Design review of the part shown in the three views and the two pictorial views. Dimensions are in mm from the part's minimum x, y and z. Coordinates: 2 decimals unless noted, no trailing zeros. Write each loop counter-clockwise with the first axis right and the second up, starting at its lowest first coordinate (ties: lowest second). Pieces come first, ordered by that corner, then holes. Notation, with made-up numbers: (76.25, 31.5) - (90.25, 31.5) arc R21 cw to (90.25, 38.5) - close; hole circle Ø7 at (42.5, 75). An arc over 180 degrees is marked (long way). Answer as CSV lines item,"result". Start each with the question number.
Q1. We need section A-A (y = 0.6). Write out the cut boundary in (x, z) (1 decimal).
Q2. Clearance check with a flat-ended pin moving along its axis: pin 1 (3 mm diameter, centred on x = 7, y = 2.5, fed in from +Z). State where the tip first meets the part, or that it passes through.
Q3. We need section B-B (y = 1.65). Write out the cut boundary in (x, z) (1 decimal).
Q4. For line 1 along X through (y, z) = (1.4, 6); line 2 along Z through (x, y) = (9, 4.6) (1 decimal); line 3 along X through (y, z) = (0.3, 7.5) (1 decimal), list the stretches that pass through material, from the lowest coordinate up. Write a range as [from, to].
Q5. Mouldability with a two-part tool opening along X and no side actions: class the marked faces 1, 2 and 3 as pulls with the +X half, pulls with the -X half, needs draft (parallel to the pull), parting line crosses it, or undercut.
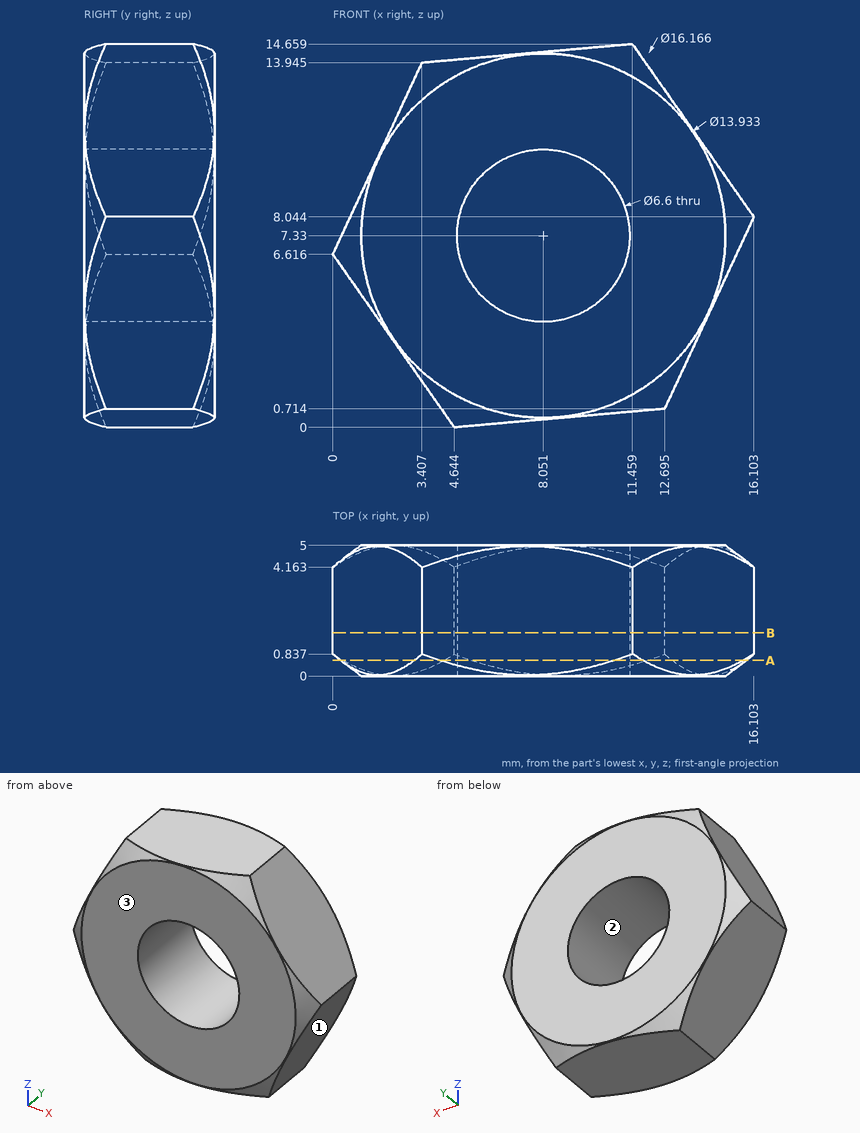
Results list:
1,outline,"(0.3, 7.2) arc R7.8 ccw to (0.4, 6.1) - (4.3, 0.6) arc R7.8 ccw to (5.3, 0.1) - (12, 0.7) arc R7.8 ccw to (13, 1.3) - (15.8, 7.4) arc R7.8 ccw to (15.7, 8.6) - (11.8, 14.1) arc R7.8 ccw to (10.8, 14.6) - (4.1, 14) arc R7.8 ccw to (3.1, 13.3) - close; hole circle Ø6.6 at (8.1, 7.3)"
2,pin 1,"stops at z = 14.4"
3,outline,"(0, 6.6) - (4.6, 0) - (12.7, 0.7) - (16.1, 8) - (11.5, 14.7) - (3.4, 13.9) - close; hole circle Ø6.6 at (8.1, 7.3)"
4,line 1,"x = [0.43, 5.03], [11.07, 15.15]"
4,line 2,"z = [0.4, 4.2], [10.5, 14.4]"
4,line 3,"x = [0.7, 4.8], [11.3, 15.4]"
5,face 1,"pulls with the +X half"
5,face 2,"undercut"
5,face 3,"needs draft"
